Input: part model. Units: mm. Frame: model coordinates. A direction names the side the tool comes from. Give positions to 0.01 mm unless a question says otherwise; leave off trailing zeros. Write each loop counter-clockwise with the first axis right and the second up, starting at its lowest first coordinate (ties: lowest second). Pieces come first, ordered by that corner, then holes. Notation, with made-up numbers: (80.25, -16) - (112.25, -16) arc R21 ccw to (112.25, -8) - close; hole circle Ø9 at (21.5, 37.25). An arc over 180 degrees is marked (long way). Answer as CSV lines item,"result". Start each with the question number.
Autodesk Inventor part; units mm, degrees
ref_plane "Work Plane1" through (17.4625, -12.7, 0) normal (1, 0, 0) x (0, 0, -1)
ref_plane "YZ Plane" through (0, 0, 0) normal (1, 0, 0) x (0, 1, 0)
ref_plane "XZ Plane" through (0, 0, 0) normal (0, 1, 0) x (-1, 0, 0)
sketch "Sketch1" plane through (0, 0, 0) normal (0, 0, 1) x (1, 0, 0)
  line L0 (-12.7, -12.7) -> (12.7, -12.7)
  line L1 (12.7, -12.7) -> (12.7, 12.7)
  line L2 (12.7, 12.7) -> (-12.7, 12.7)
  line L3 (-12.7, 12.7) -> (-12.7, -12.7)
  line L4 (-12.7, -12.7) -> (12.7, 12.7) construction
  line L5 (12.7, -12.7) -> (-12.7, 12.7) construction
  line L6 (9.525, -9.525) -> (-9.525, -9.525)
  line L7 (-9.525, -9.525) -> (-9.525, 9.525)
  line L8 (-9.525, 9.525) -> (9.525, 9.525)
  line L9 (9.525, 9.525) -> (9.525, -9.525)
  line L10 (9.525, -9.525) -> (-9.525, 9.525) construction
  line L11 (-9.525, -9.525) -> (9.525, 9.525) construction
  point P0 (0, 0)
  dimension "d0" = 25.4
  dimension "d1" = 25.4
  dimension "d6" = 3.175
  dimension "d7" = 3.175
extrude "Extrusion1" add sketch "Sketch1" along normal blind 660.4
sketch "Sketch2" plane through (-12.7, -12.7, 0) normal (-1, 0, 0) x (0, 0, 1)
  line L0 (95.377, -0.127) -> (131.064, -0.127)
  line L1 (131.064, -0.127) -> (133.223, 2.032)
  line L2 (133.223, 2.032) -> (133.223, 23.114)
  line L3 (133.223, 23.114) -> (131.064, 25.273)
  line L4 (131.064, 25.273) -> (65.786, 25.273)
  line L5 (65.786, 25.273) -> (63.627, 23.114)
  line L6 (63.627, 23.114) -> (63.627, -42.164)
  line L7 (63.627, -42.164) -> (65.786, -44.323)
  line L8 (65.786, -44.323) -> (86.868, -44.323)
  line L9 (86.868, -44.323) -> (89.027, -42.164)
  line L10 (89.027, -6.477) -> (89.027, -42.164)
  arc A0 (95.377, -0.127) -> (89.027, -6.477) centre (95.377, -6.477) ccw
  circle A1 centre (127, 12.7) radius 2.0701
  circle A2 centre (76.2, -25.4) radius 2.0701
  circle A3 centre (76.2, 0) radius 2.0701
  circle A4 centre (101.6, 12.7) radius 2.0701
  circle A5 centre (76.2, 12.7) radius 2.0701
  circle A6 centre (88.9, 12.7) radius 2.0701
  circle A7 centre (114.3, 12.7) radius 2.0701
  circle A8 centre (76.2, -12.7) radius 2.0701
  circle A9 centre (76.2, -38.1) radius 2.0701
  line L11 (527.177, 2.032) -> (527.177, 23.114)
  line L12 (527.177, 2.032) -> (529.336, -0.127)
  line L13 (565.023, -0.127) -> (529.336, -0.127)
  arc A10 (571.373, -6.477) -> (565.023, -0.127) centre (565.023, -6.477) ccw
  line L14 (571.373, -6.477) -> (571.373, -42.164)
  line L15 (571.373, -42.164) -> (573.532, -44.323)
  line L16 (594.614, -44.323) -> (573.532, -44.323)
  line L17 (594.614, -44.323) -> (596.773, -42.164)
  line L18 (596.773, 23.114) -> (596.773, -42.164)
  line L19 (596.773, 23.114) -> (594.614, 25.273)
  line L20 (529.336, 25.273) -> (594.614, 25.273)
  line L21 (529.336, 25.273) -> (527.177, 23.114)
  circle A11 centre (533.4, 12.7) radius 2.0701
  circle A12 centre (584.2, -25.4) radius 2.0701
  circle A13 centre (584.2, 0) radius 2.0701
  circle A14 centre (558.8, 12.7) radius 2.0701
  circle A15 centre (584.2, 12.7) radius 2.0701
  circle A16 centre (571.5, 12.7) radius 2.0701
  circle A17 centre (546.1, 12.7) radius 2.0701
  circle A18 centre (584.2, -12.7) radius 2.0701
  circle A19 centre (584.2, -38.1) radius 2.0701
  point P0 (0, 12.7)
hole "Hole1" at (-12.7, 0, 127) at (-12.7, 0, 114.3) at (-12.7, 0, 101.6) at (-12.7, 0, 88.9) at (-12.7, 0, 76.2) at (-12.7, 0, 584.2) at (-12.7, 0, 571.5) at (-12.7, 0, 558.8) at (-12.7, 0, 546.1) at (-12.7, 0, 533.4) direction (1, 0, 0) diameter 4.1402 end through all
sketch "Sketch7" plane through (0, 0, 0) normal (0, 0, -1) x (-1, 0, 0)
  line L0 (9.525, 9.525) -> (9.525, -9.525)
  line L1 (9.525, -9.525) -> (-9.525, -9.525)
  line L2 (-9.525, -9.525) -> (-9.525, 9.525)
  line L3 (-9.525, 9.525) -> (9.525, 9.525)
  line L4 (-12.7, 12.7) -> (12.7, 12.7)
  line L5 (-11.1125, -11.1125) -> (11.1125, -11.1125)
  line L6 (11.1125, -11.1125) -> (11.1125, 11.1125)
  line L7 (11.1125, 11.1125) -> (-11.1125, 11.1125)
  line L8 (-11.1125, 11.1125) -> (-11.1125, -11.1125)
  line L9 (-11.1125, -11.1125) -> (11.1125, 11.1125) construction
  line L10 (11.1125, -11.1125) -> (-11.1125, 11.1125) construction
  point P0 (0, 0)
  dimension "d33" = 1.5875
extrude "Extrusion5" cut sketch "Sketch7" against normal through all
ref_plane "Work Plane1" through (17.4625, -12.7, 0) normal (1, 0, 0) x (0, 0, -1)
sketch "Sketch9" plane through (12.7, -12.7, 0) normal (1, 0, 0) x (0, 0, -1)
  line L0 (-660.4, 25.4) -> (-596.9, 25.4)
  line L1 (-596.9, 25.4) -> (-596.9, 0)
  line L2 (-596.9, 0) -> (-660.4, 0)
  line L3 (-660.4, 0) -> (-660.4, 25.4)
  line L4 (0, 25.4) -> (-63.5, 25.4)
  line L5 (-63.5, 25.4) -> (-63.5, 0)
  line L6 (-63.5, 0) -> (0, 0)
  line L7 (0, 0) -> (0, 25.4)
  line L8 (0, 0) -> (-660.4, 0)
  point P0 (0, 12.7)
  dimension "d42" = 63.5
  dimension "d43" = 63.5
extrude "Extrusion7" cut sketch "Sketch9" against normal through all
properties part number "C24R2_TK_ShooterPivotStock"
1) Material intervals for line 1 (X direction, y = 10, z = 229); line 2 (Y direction, x = -11.65, z = 571.5), sorted ascending. Write a range as from..to.
2) Pull-direction query (Y, two-part tool) for faces 1 (the flat face through (11.112, 0, 326)), 2 (the flat face through (0, 12.7, 326)), 3 (the flat face through (0, -12.7, 326)); classes: +Y half, -Y half, draft (parallel to the pull), parting line (faces both ways), or undercut.
3) Cut plane A-A on y = 6. Output: boundary loops of the cut face in (x, z).
4) Cut plane B-B on z = 287. Output: boundary loops of the cut face in (x, y), and give its area (3 significant figures).
5) Reachability of faces 4 (the flat face through (-12.7, 0, 326)), 5 (the flat face through (-11.112, 0, 326)) from +Z, -Z, +X, -X, +Y, -Y: full face, straight path, thin tool, end or side. Return the list, or none.
6) Contact query for flat-ended pins moving along their axis: P1, Ø5, axis at y = 0, z = 127, coming from the +X side; P2, Ø3.5, axis at y = 0, z = 558.8, coming from the +X side. Output: stop coordinate, or through.
Numbers:
1,line 1,"x = -12.7..-11.11, 11.11..12.7"
1,line 2,"y = -12.7..-2.07, 2.07..12.7"
2,face 1,"undercut"
2,face 2,"+Y half"
2,face 3,"-Y half"
3,outline,"(-12.7, 63.5) - (-11.11, 63.5) - (-11.11, 596.9) - (-12.7, 596.9) - close; (11.11, 63.5) - (12.7, 63.5) - (12.7, 596.9) - (11.11, 596.9) - close"
4,outline,"(-12.7, -12.7) - (12.7, -12.7) - (12.7, 12.7) - (-12.7, 12.7) - close; hole (-11.11, -11.11) - (11.11, -11.11) - (11.11, 11.11) - (-11.11, 11.11) - close"
4,area,"151 mm²"
5,face 4,"+Z, -Z, -X, +Y, -Y"
5,face 5,"+Z, -Z"
6,P1,"stops at x = 12.7"
6,P2,"passes through"
